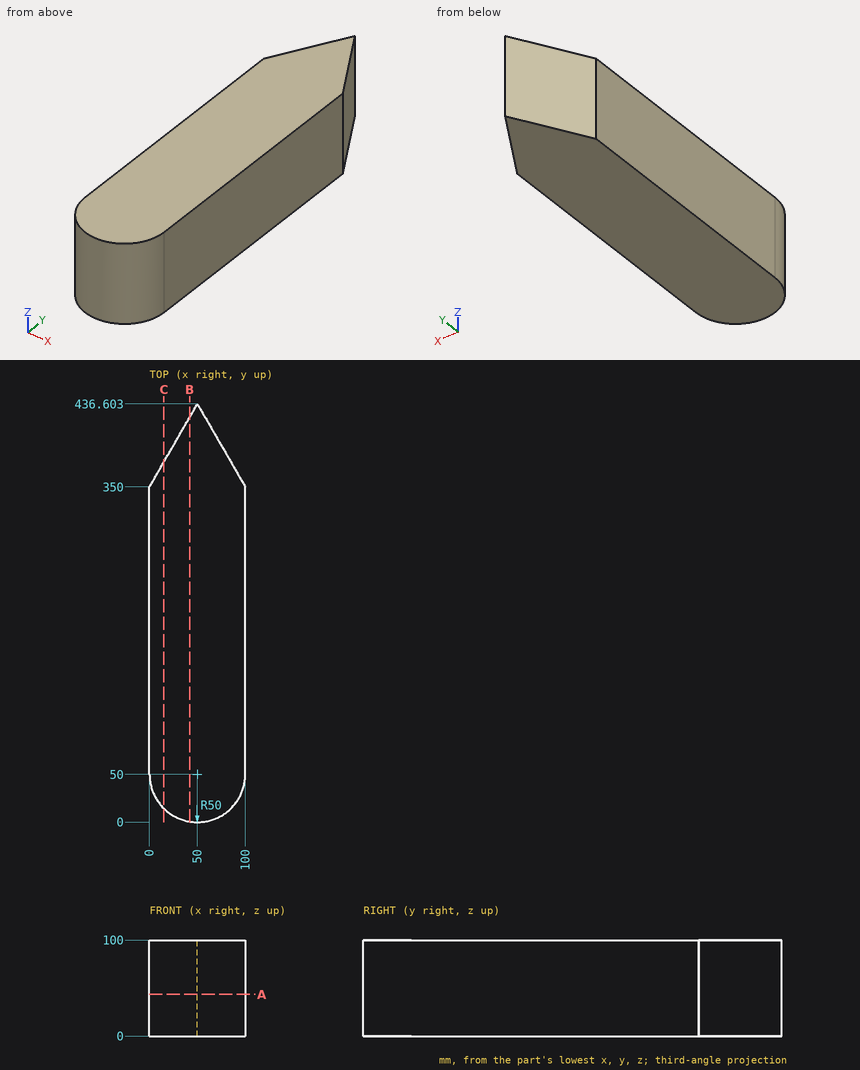
Part print with two shaded views. Sizes in mm from the minimum x, y, z corner. Coordinates: 2 decimals unless noted, no trailing zeros. Order: outer loops, then holes, each group sorted by start corner. A loop starts at its lowest first (then second) coordinate and runs counter-clockwise, first axis right, second up. Notation, with made-up numbers: M -37,87.25 L -22,87.25 A22 cw -22,113.25 Z; hole C 59,24 d9. An arc over 180 degrees is marked long. Use a Markdown table: item, result.
(1) Cut at B-B on x = 42. Write the cut outline in (y, z) (1 decimal).
A:
| item | result |
|---|---|
| outline | M 0.6,0 L 422.7,0 L 422.7,100 L 0.6,100 Z |
(2) Cut at A-A on z = 43.5. Write the cut outline in (x, y), then the cut area to 3 significant figures.
A:
| item | result |
|---|---|
| outline | M 0,50 A50 ccw 100,50 L 100,350 L 50,436.6 L 0,350 Z |
| area | 38,300 mm^2 |
(3) Cut at C-C on x = 15. Write the cut outline in (y, z).
A:
| item | result |
|---|---|
| outline | M 14.29,0 L 375.98,0 L 375.98,100 L 14.29,100 Z |
(4) Flat gauge pins, fed straight in: pin 1 (10 mm diameter, centred on x = 15.5, z = 39.5, fed in from +Y) (1 decimal); pin 2 (1.5 mm diameter, centred on x = 59, z = 10.5, fed in from -Y) (1 decimal); pin 3 (2 mm diameter, centred on x = 42, z = 40, fed in from +Y). Where does each tip first touch, or does it go through?
A:
| item | result |
|---|---|
| pin 1 | stops at y = 385.5 |
| pin 2 | stops at y = 0.7 |
| pin 3 | stops at y = 424.48 |
(5) Probe L1, parallel to Y at x = 42.5, z = 63 (1 decimal); L2, parallel to X at y = 391.5, z = 63.5; L3, parallel to Y at x = 50.5, z = 22.5 (1 decimal). List the from-to ranges inside material, lowest first.
A:
| item | result |
|---|---|
| L1 | y = 0.6 to 423.6 |
| L2 | x = 23.96 to 76.04 |
| L3 | y = 0 to 435.7 |
